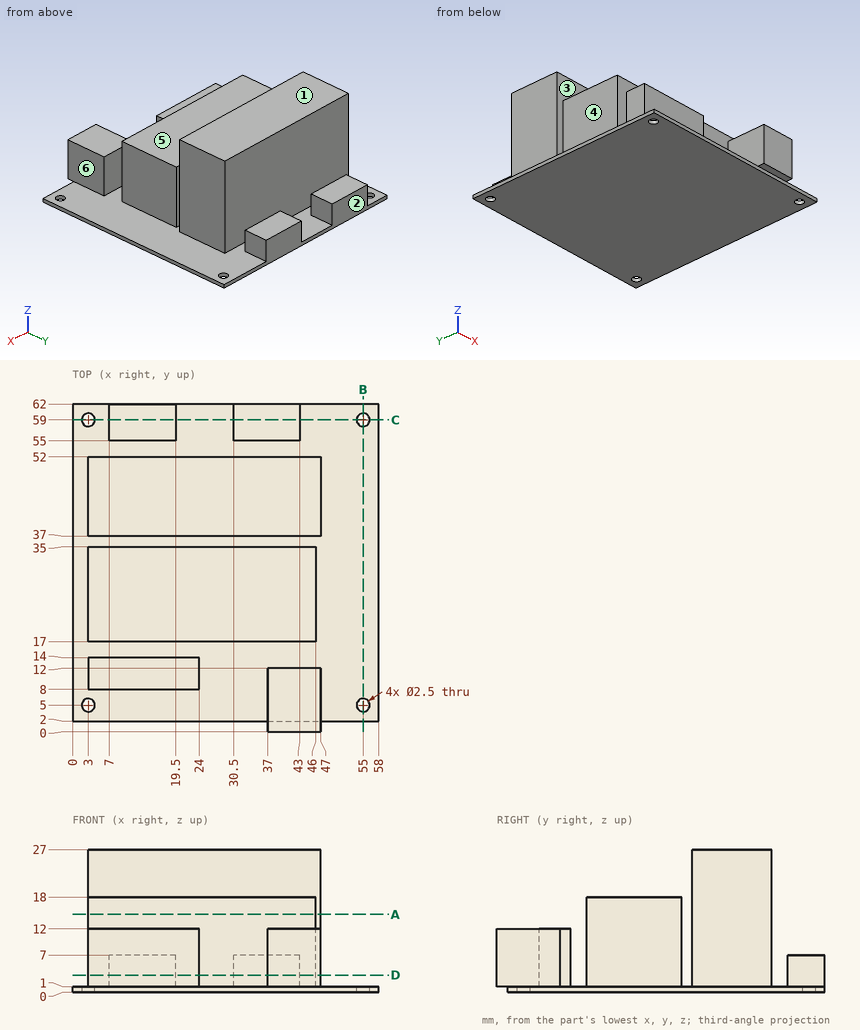
Verification items for this drawing (mm, ordinates from the low corner). A direction names the side the tool comes from. Coordinates: 2 decimals unless noted, no trailing zeros. Order: outer loops, then holes, each group sorted by start corner. A loop starts at its lowest first (then second) coordinate and runs counter-clockwise, first axis right, second up. Notation, with made-up numbers: M 43,-19.5 L 74,-19.5 A6 cw 74,-13.5 Z; hole C 13.5,-18.5 d3. An arc over 180 degrees is marked long. Answer as a JSON object with one key per item and string values.
Q1. Tool access check on the marked faces 4, 5 and 6. Record the directions out of +Z, -Z, +X, -X, +Y, -Y that give a thin tool (end or side, any length) a straight path to the whole face; none if there is none.
Results are:
{"face 4": "+Z, -X, +Y, -Y", "face 5": "+Z, +X, -X, -Y", "face 6": "+Z, +X, +Y, -Y"}
Q2. Depth check by flat-ended pin: pin 1 Ø1 at (y, z) = (44, 7.5) entering from +X; pin 2 Ø12 at (x, z) = (44, 13) entering from +Y; pin 3 Ø6.5 at (y, z) = (9.5, 4.5) entering from -X. Enter the tip coordinate at first touch or a pass-through.
Results are:
{"pin 1": "stops at x = 47", "pin 2": "stops at y = 52", "pin 3": "stops at x = 3"}
Q3. Scan lines: line 1 (Y direction, x = 12, z = 2.25); line 2 (Y direction, x = 3, z = 0.5); line 3 (Y direction, x = 15, z = 10). Record each from-to range of solid material in increasing order.
Results are:
{"line 1": "y = 8 to 14, 17 to 35, 37 to 52, 55 to 62", "line 2": "y = 2 to 3.75, 6.25 to 57.75, 60.25 to 62", "line 3": "y = 8 to 14, 17 to 35, 37 to 52"}
Q4. Cross-section at C-C on y = 59. Record the cut outline in (x, z), and give its area (3 significant figures).
Results are:
{"outline": "M 0,0 L 1.75,0 L 1.75,1 L 0,1 Z; M 4.25,0 L 53.75,0 L 53.75,1 L 43,1 L 43,7 L 30.5,7 L 30.5,1 L 19.5,1 L 19.5,7 L 7,7 L 7,1 L 4.25,1 Z; M 56.25,0 L 58,0 L 58,1 L 56.25,1 Z", "area": "203 mm²"}
Q5. Release check for a two-part mould opening along Y. For the marked faces 1, 2 and 3 record: released by +Y, released by -Y, zero draft, split by the parting line, or undercut.
Results are:
{"face 1": "zero draft", "face 2": "released by +Y", "face 3": "undercut"}
Q6. Cross-section at B-B on x = 55. Record the cut outline in (y, z), and give its area (3 significant figures).
Results are:
{"outline": "M 2,0 L 3.75,0 L 3.75,1 L 2,1 Z; M 6.25,0 L 57.75,0 L 57.75,1 L 6.25,1 Z; M 60.25,0 L 62,0 L 62,1 L 60.25,1 Z", "area": "55.0 mm²"}
Q7. Cross-section at D-D on z = 3.25. Record the cut outline in (x, y).
Results are:
{"outline": "M 3,8 L 24,8 L 24,14 L 3,14 Z; M 3,17 L 46,17 L 46,35 L 3,35 Z; M 3,37 L 47,37 L 47,52 L 3,52 Z; M 7,55 L 19.5,55 L 19.5,62 L 7,62 Z; M 30.5,55 L 43,55 L 43,62 L 30.5,62 Z; M 37,0 L 47,0 L 47,12 L 37,12 Z"}
Q8. Cross-section at A-A on z = 14.75. Record the cut outline in (x, y), and give its area (3 significant figures).
Results are:
{"outline": "M 3,17 L 46,17 L 46,35 L 3,35 Z; M 3,37 L 47,37 L 47,52 L 3,52 Z", "area": "1,430 mm²"}
